Part model, mm, in its own coordinate system. A direction names the side the tool comes from. Round coordinates to 2 decimals unless told otherwise and drop trailing zeros. Write each loop counter-clockwise with the first axis right and the second up, starting at its lowest first coordinate (ties: lowest second). Pieces come first, ordered by that corner, then holes.
```python
from build123d import *

# Parameters (mm, degrees)
F1_DEPTH = 10
F2_SIZE2 = 1
F2_SIZE  = 1
F3_R     = 8
F4_DEPTH = 40
F5_R     = 8
F5_R_2   = 7.9
F6_DEPTH = 38


with BuildPart() as f1:
    # F0 (on Front) → F1 (new body)
    with BuildSketch(Plane.XZ):
        Polygon((0, -13.856406), (12, -6.928203), (12, 6.928203), (0, 13.856406), (-12, 6.928203), (-12, -6.928203), align=None)
    extrude(amount=F1_DEPTH)

    # F2
    f2_edges = [f1.edges().sort_by_distance(p)[0] for p in [
        (6, -10, 10.392305),
        (-6, -10, 10.392305),
        (12, -10, 0),
        (6, -10, -10.392305),
        (-6, -10, -10.392305),
        (-12, -10, 0),
    ]]
    chamfer(f2_edges, length=F2_SIZE, length2=F2_SIZE2)

    # F3 (on face) → F4 (join)
    with BuildSketch(Plane(origin=(0, 0, 0), x_dir=(-1, 0, 0), z_dir=(0, 1, 0))):
        Circle(F3_R)
    extrude(amount=F4_DEPTH)

    # F5 (on face) → F6 (cut)
    with BuildSketch(Plane(origin=(0, 40, 0), x_dir=(-1, 0, 0), z_dir=(0, 1, 0))):
        Circle(F5_R)
        Circle(F5_R_2, mode=Mode.SUBTRACT)
    extrude(amount=-F6_DEPTH, mode=Mode.SUBTRACT)


solid = f1.part
```
Q1. Wall check: L1, parallel to Y at x = -8.5, z = 3.5; L2, parallel to Z at x = -6, y = -6; L3, parallel to Z at x = -5, y = -1. Give the ranges that are in metal, low to high.
Values follow:
L1: y = -10 to 0
L2: z = -10.39 to 10.39
L3: z = -10.97 to 10.97
Q2. Drop flat-ended pins along their axis: pin 1 (5 mm diameter, centred on x = -1.5, y = 3, fed in from -Z); pin 2 (2 mm diameter, centred on y = 10.5, z = 0.5, fed in from +X); pin 3 (12 mm diameter, centred on x = -4, y = 11.5, fed in from -Z). Give the stop position or say it passes through.
Values follow:
pin 1: stops at z = -8
pin 2: stops at x = 7.9
pin 3: stops at z = -7.9
Q3. Which spindle directions (+Z, -Z, +X, -X, +Y, -Y) get a long thin tool onto all of the face, cutting with end or side? Do faces 1 (the flat face through (-12, -4, 0)), 2 (the flat face through (-6, 0, -6)). Say none if no direction does.
Values follow:
face 1: +Z, -Z, -X, +Y, -Y
face 2: +Y
Q4. Cut at C-C on y = -5.5. Write the cut outline in (x, z), plus the area to 3 significant figures.
Values follow:
outline: (-12, -6.93) - (0, -13.86) - (12, -6.93) - (12, 6.93) - (0, 13.86) - (-12, 6.93) - close
area: 499 mm2
Q5. Cut at D-D on x = -10.25. Write the cut outline in (y, z).
Values follow:
outline: (-10, -6.78) - (-9, -7.94) - (0, -7.94) - (0, 7.94) - (-9, 7.94) - (-10, 6.78) - close
Q6. Cut at A-A on z = 0. Write the cut outline in (x, y).
Values follow:
outline: (-12, -9) - (-11, -10) - (11, -10) - (12, -9) - (12, 0) - (8, 0) - (8, 2) - (7.9, 2) - (7.9, 40) - (-7.9, 40) - (-7.9, 2) - (-8, 2) - (-8, 0) - (-12, 0) - close
Q7. Cut at B-B on x = -4.75. Write the cut outline in (y, z), plus the area to 3 significant figures.
Values follow:
outline: (-10, -9.96) - (-9, -11.11) - (0, -11.11) - (0, -6.44) - (2, -6.44) - (2, -6.31) - (40, -6.31) - (40, 6.31) - (2, 6.31) - (2, 6.44) - (0, 6.44) - (0, 11.11) - (-9, 11.11) - (-10, 9.96) - close
area: 727 mm2
